Autodesk Inventor part; units mm, degrees
ref_plane "YZ Plane" through (0, 0, 0) normal (1, 0, 0) x (0, 1, 0)
ref_plane "XZ Plane" through (0, 0, 0) normal (0, 1, 0) x (-1, 0, 0)
ref_plane "XY Plane" through (0, 0, 0) normal (0, 0, 1) x (1, 0, 0)
sketch "Эскиз1" plane through (0, 0, 0) normal (0, 1, 0) x (-1, 0, 0)
  circle A0 centre (0, 0) radius 9.1
  line L0 (0, -10.7442) -> (-9.3048, -5.3721)
  line L1 (-9.3048, -5.3721) -> (-9.3048, 5.3721)
  line L2 (-9.3048, 5.3721) -> (0, 10.7442)
  line L3 (0, 10.7442) -> (9.3048, 5.3721)
  line L4 (9.3048, 5.3721) -> (9.3048, -5.3721)
  line L5 (9.3048, -5.3721) -> (0, -10.7442)
  circle A1 centre (0, 0) radius 9.3048
  dimension "d0" = 18.2
extrude "Выдавливание1" add sketch "Эскиз1" along normal blind 10 contours A1
properties part number "18650"
Could you check a few things on this model? Use its own coordinates, in mm. Give positions to 0.01 mm unless a question says otherwise; leave off trailing zeros. Loops run counter-clockwise (first coordinate to the right, second up) from the corner with the lowest first, then second, coordinate; pieces in that order, holes last. Notation, with made-up numbers: (51, -5) -> (83, -5) arc R19 cw to (83, 19) -> close; hole circle Ø9 at (62.25, 0.5). An arc over 180 degrees is marked (long way). Answer as CSV lines item,"result". Start each with the question number.
(1) If we section it at C-C on y = 9: Write out the boundary of the cut face in (x, z).
(2) I need wall thicknesses on probe 1 along Z at (x, y) = (0, 4.5); probe 2 along Z at (x, y) = (3.25, 7.5); probe 3 along X at (y, z) = (5.5, 8.25). Which ranges of each line are inside material? Lowest first, please.
(3) If we section it at A-A on z = 0: Write out the boundary of the cut face in (x, y), then the cut area to 3 significant figures.
(4) I'm going to push flat-ended pins straight in: pin 1 Ø1 at (x, z) = (-7, 3) entering from +Y; pin 2 Ø1 at (y, z) = (4, 7.5) entering from -X; pin 3 Ø4 at (y, z) = (1.5, -6.5) entering from -X. Where does each tip first touch, or does it pass through?
(5) If we section it at B-B on x = 0: Write out the boundary of the cut face in (y, z), then the cut area to 3 significant figures.
(6) We'd pull the mould along Z, two halves only. Please class faces 1 (the cylindrical face through (2.017, 4.93, 9.084)), 2 (the cylindrical face through (1.973, 4.93, 8.884)): released by +Z, released by -Z, zero draft, split by the parting line, or undercut.
Computed:
1,outline,"circle Ø18.61 at (0, 0); hole circle Ø18.2 at (0, 0)"
2,probe 1,"z = -9.3 to -9.1, 9.1 to 9.3"
2,probe 2,"z = -8.72 to -8.5, 8.5 to 8.72"
2,probe 3,"x = -4.3 to -3.84, 3.84 to 4.3"
3,outline,"(-9.3, 0) -> (-9.1, 0) -> (-9.1, 10) -> (-9.3, 10) -> close; (9.1, 0) -> (9.3, 0) -> (9.3, 10) -> (9.1, 10) -> close"
3,area,"4.10 mm2"
4,pin 1,"passes through"
4,pin 2,"stops at x = -6.13"
4,pin 3,"stops at x = -8.14"
5,outline,"(0, -9.3) -> (10, -9.3) -> (10, -9.1) -> (0, -9.1) -> close; (0, 9.1) -> (10, 9.1) -> (10, 9.3) -> (0, 9.3) -> close"
5,area,"4.10 mm2"
6,face 1,"split by the parting line"
6,face 2,"undercut"
